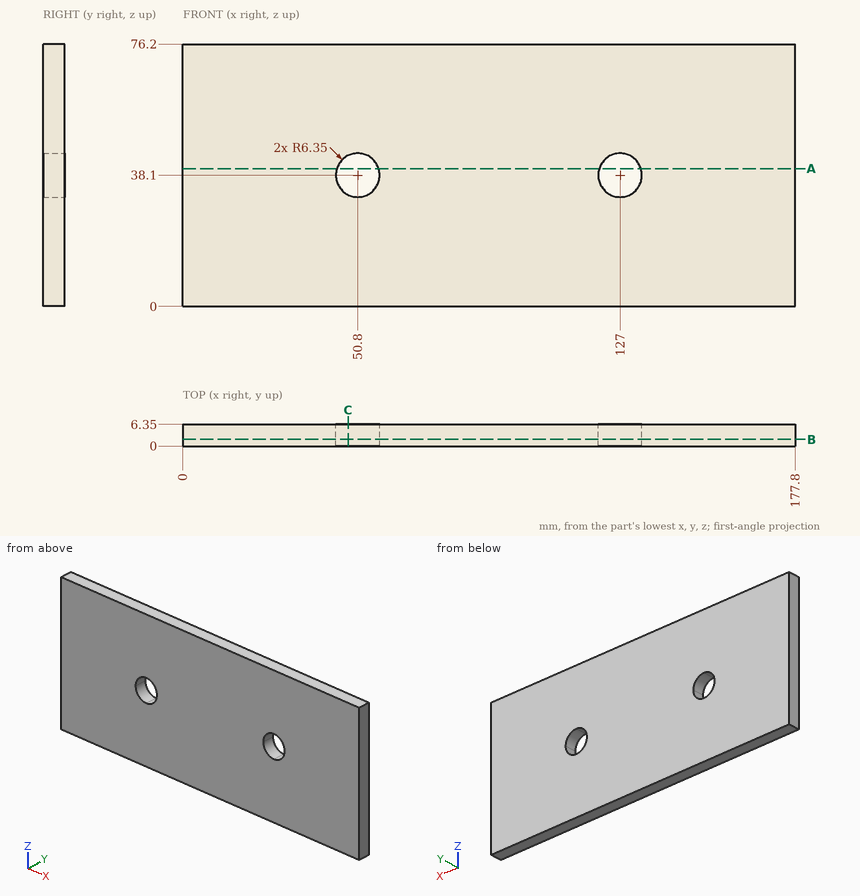
Check sheet for the drawn part. Datum: minimum x, y, z corner. Units: mm. Round coordinates to 2 decimals unless told otherwise and drop trailing zeros. Write each loop counter-clockwise with the first axis right and the second up, starting at its lowest first coordinate (ties: lowest second). Pieces come first, ordered by that corner, then holes. Notation, with made-up numbers: (73, 2.5) -> (121, 2.5) arc R11 cw to (121, 15.5) -> close; hole circle Ø5 at (25, 1). An arc over 180 degrees is marked (long way). Write each question's results on one line, items separated by ' | '. Start each with the question number.
1. Material ranges on probe 1 along Z at (x, y) = (127, 1); probe 2 along X at (y, z) = (2.5, 36.5); probe 3 along X at (y, z) = (3.5, 43), recorded low to high. Write a range as from..to.
2. Depth check by flat-ended pin: P1, Ø5, axis at x = 55, z = 14.5, coming from the -Y side. Enter the tip coordinate at first touch or a pass-through.
3. Cross-section at A-A (z = 40). Enter the section's corners in (x, y), then the cut area to 3 significant figures.
4. Cross-section at B-B (y = 2). Enter the section's corners in (x, z).
5. Cross-section at C-C (x = 48). Enter the section's corners in (y, z), then the cut area to 3 significant figures.
Solutions:
1) probe 1: z = 0..31.75, 44.45..76.2 | probe 2: x = 0..44.65, 56.95..120.85, 133.15..177.8 | probe 3: x = 0..46.76, 54.84..122.96, 131.04..177.8
2) P1: stops at y = 0
3) outline: (0, 0) -> (44.74, 0) -> (44.74, 6.35) -> (0, 6.35) -> close; (56.86, 0) -> (120.94, 0) -> (120.94, 6.35) -> (56.86, 6.35) -> close; (133.06, 0) -> (177.8, 0) -> (177.8, 6.35) -> (133.06, 6.35) -> close | area: 975 mm2
4) outline: (0, 0) -> (177.8, 0) -> (177.8, 76.2) -> (0, 76.2) -> close; hole circle Ø12.7 at (50.8, 38.1); hole circle Ø12.7 at (127, 38.1)
5) outline: (0, 0) -> (6.35, 0) -> (6.35, 32.4) -> (0, 32.4) -> close; (0, 43.8) -> (6.35, 43.8) -> (6.35, 76.2) -> (0, 76.2) -> close | area: 411 mm2
